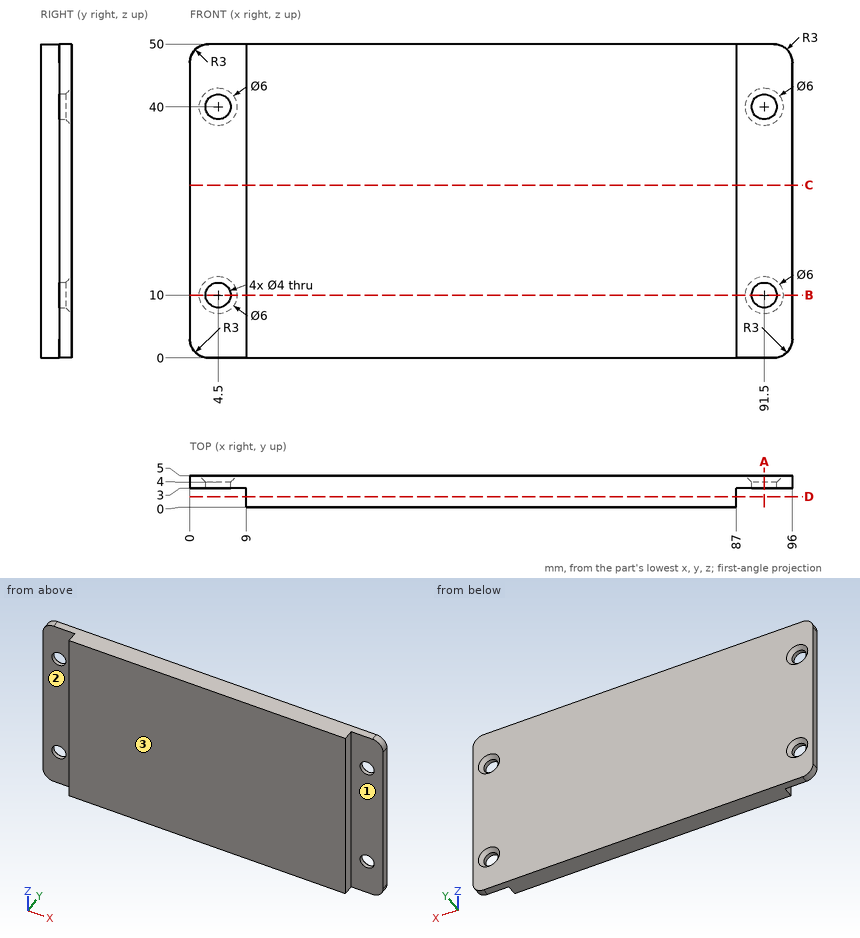
Geometry: see drawing. Coordinates: mm, zero at the bounding-box minimum. A direction names the side the tool comes from. Coordinates: 2 decimals unless noted, no trailing zeros. Write each loop counter-clockwise with the first axis right and the second up, starting at its lowest first coordinate (ties: lowest second). Pieces come first, ordered by that corner, then holes. Notation, with made-up numbers: M -31,-0.5 L 10,-0.5 A13 ccw 10,3.5 Z; hole C -29.75,55 d8. An arc over 180 degrees is marked long. Use CSV: the item, a comma, the result in double quotes. Start each with the question number.
1. Cut plane C-C on z = 27.5. Return the cut outline in (x, y), plus the area to 3 significant figures.
2. Cut plane A-A on x = 91.5. Return the cut outline in (y, z), plus the area to 3 significant figures.
3. Cut plane D-D on y = 1.7. Return the cut outline in (x, z), plus the area to 3 significant figures.
4. Ray query, probe 1 along X at (y, z) = (3.4, 10); probe 2 along X at (y, z) = (2.05, 41). Return the intervals inside material, ascending.
5. Reachability of the marked faces 1, 2 and 3 from +Z, -Z, +X, -X, +Y, -Y: full face, straight path, thin tool, end or side. Return the list, or none.
6. First-contact query: P1, Ø3, axis at x = 4.5, z = 10, coming from the -Y side; P2, Ø2.5, axis at x = 3, z = 24, coming from the -Y side; P3, Ø1.5, axis at y = 2, z = 23.5, coming from the +X side. Flat tips, straight axial feed; report the tip coordinate or a pass-through.
7. Cut plane B-B on z = 10. Return the cut outline in (x, y).
Entries:
1,outline,"M 0,3 L 9,3 L 9,0 L 87,0 L 87,3 L 96,3 L 96,5 L 0,5 Z"
1,area,"426 mm²"
2,outline,"M 3,0 L 5,0 L 5,7 L 4,8 L 3,8 Z; M 3,12 L 4,12 L 5,13 L 5,37 L 4,38 L 3,38 Z; M 3,42 L 4,42 L 5,43 L 5,50 L 3,50 Z"
2,area,"82.0 mm²"
3,outline,"M 9,0 L 87,0 L 87,50 L 9,50 Z"
3,area,"3,900 mm²"
4,probe 1,"0 to 2.5, 6.5 to 89.5, 93.5 to 96"
4,probe 2,"9 to 87"
5,face 1,"+Z, -Z, +X, -Y"
5,face 2,"+Z, -Z, -X, -Y"
5,face 3,"+Z, -Z, +X, -X, -Y"
6,P1,"through"
6,P2,"y = 3"
6,P3,"x = 87"
7,outline,"M 0,3 L 2.5,3 L 2.5,4 L 1.5,5 L 0,5 Z; M 6.5,3 L 9,3 L 9,0 L 87,0 L 87,3 L 89.5,3 L 89.5,4 L 88.5,5 L 7.5,5 L 6.5,4 Z; M 93.5,3 L 96,3 L 96,5 L 94.5,5 L 93.5,4 Z"
